from build123d import *

# Parameters (mm, degrees)
SKETCH1_W                    = 57.15
SKETCH1_H                    = 38.1
BASE_FLANGE1_DEPTH           = 1.89738
EDGE_FLANGE1_STRIP_W         = 11.38428
EDGE_FLANGE1_STRIP_H         = 1.89738
EDGE_FLANGE1_STRIP_CUT_DEPTH = 57.15
EDGE_FLANGE1_DEPTH           = 57.15
F_1_4_CLEARANCE_HOLE1_D      = 6.7564
F_1_4_CLEARANCE_HOLE2_D      = 6.7564
FILLET1_R                    = 6.35


# Sheet-metal steps are written as plain solids
with BuildPart() as part:
    # Sketch1 → Base-Flange1 (new body)
    with BuildSketch(Plane(origin=(0, 0, 0), x_dir=(1, 0, 0), z_dir=(0, 1, 0))):
        with Locations((0, -19.05)):
            Rectangle(SKETCH1_W, SKETCH1_H)
    extrude(amount=BASE_FLANGE1_DEPTH)

    # Edge-Flange1 strip (across the edge) → Edge-Flange1 strip cut (cut)
    with BuildSketch(Plane(origin=(28.575, 1.89738, 0), x_dir=(0, 0, 1), z_dir=(-1, 0, 0))):
        with Locations((-1.89738, -0.94869)):
            Rectangle(EDGE_FLANGE1_STRIP_W, EDGE_FLANGE1_STRIP_H)
    extrude(amount=EDGE_FLANGE1_STRIP_CUT_DEPTH, mode=Mode.SUBTRACT)

    # Edge-Flange1 section (across the edge) → Edge-Flange1 (add)
    with BuildSketch(Plane(origin=(28.575, 1.89738, 0), x_dir=(0, 0, 1), z_dir=(-1, 0, 0))):
        with BuildLine():
            Line((0, 1.89738), (0, 36.20262))
            Line((0, 36.20262), (1.89738, 36.20262))
            Line((1.89738, 36.20262), (1.89738, 1.89738))
            ThreePointArc((1.89738, 1.89738), (2.453109736, 0.555729736), (3.79476, 0))
            Line((3.79476, 0), (3.79476, -1.89738))
            ThreePointArc((3.79476, -1.89738), (1.111459471, -0.785920529), (0, 1.89738))
        make_face()
    extrude(amount=EDGE_FLANGE1_DEPTH)

    # 1/4 Clearance Hole1 (through all)
    with Locations(Plane(origin=(0, 1.89738, 0), x_dir=(1, 0, 0), z_dir=(0, 1, 0))):
        with Locations((-15.875, -25.4), (15.875, -25.4)):
            Hole(F_1_4_CLEARANCE_HOLE1_D / 2)

    # 1/4 Clearance Hole2 (through all)
    with Locations(Plane.XY.offset(1.89738)):
        with Locations((-15.875, 25.4), (15.875, 25.4)):
            Hole(F_1_4_CLEARANCE_HOLE2_D / 2)

    # Fillet1
    fillet1_edges = [part.edges().sort_by_distance(p)[0] for p in [
        (28.575, 38.1, 0.94869),
        (-28.575, 38.1, 0.94869),
        (28.575, 0.94869, 38.1),
        (-28.575, 0.94869, 38.1),
    ]]
    fillet(fillet1_edges, radius=FILLET1_R)


solid = part.part
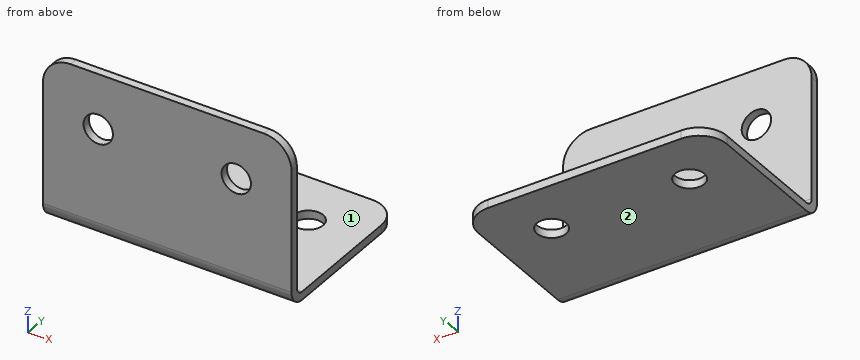
Read the model definition and answer for the solid it produces. Units are mm, in the model's axes. Face numbers are marked on the shaded views. A direction names the side the tool comes from. Round coordinates to 2 decimals unless told otherwise and drop trailing zeros. Order: outer loops, then holes, each group sorted by start corner. A loop starts at its lowest first (then second) coordinate and runs counter-clockwise, first axis right, second up.
1) For the marked faces 1 and 2, determine the directions among +Z, -Z, +X, -X, +Y, -Y from which every point of the face is accessible in a straight line to the end or side of a thin tool.
2) Flat-ended cylindrical pins translate along their axes: pin 1 (5 mm diameter, centred on x = 8, y = 29.5, fed in from +Z); pin 2 (4 mm diameter, centred on x = 21.5, z = 29.5, fed in from +Y). Find the tip coordinate at first contact, or state that the pin passes through.
3) Straight lines are drawn through the part: L1, parallel to Y at x = 12.5, z = 23; L2, parallel to Z at x = 0, y = 3. For each, find the intervals that lie inside material, in ascending order.
4) The part is cut by section C-C on x = 11.5. Write down the section's boundary in (y, z).
5) The part is cut by section A-A on y = 25.4. Write down the section's boundary in (x, z) (3 decimals).
6) The part is cut by section D-D on z = 19.5. Write down the section's boundary in (x, y) (3 decimals), plus the area to 3 significant figures.
Resolved:
1. face 1: +Z, +X, -X, +Y
1. face 2: -Z, +X, -X, +Y, -Y
2. pin 1: stops at z = 1.9
2. pin 2: stops at y = 1.9
3. L1: y = 0 to 1.9
3. L2: z = 0.08 to 2.07
4. outline: (0, 3.79) arc R3.79 ccw to (3.79, 0) - (38.1, 0) - (38.1, 1.9) - (3.79, 1.9) arc R1.9 cw to (1.9, 3.79) - (1.9, 38.1) - (0, 38.1) - close
5. outline: (-28.575, 0) - (-19.253, 0) - (-19.253, 1.897) - (-28.575, 1.897) - close; (-12.497, 0) - (12.497, 0) - (12.497, 1.897) - (-12.497, 1.897) - close; (19.253, 0) - (28.575, 0) - (28.575, 1.897) - (19.253, 1.897) - close
6. outline: (-28.575, 0) - (28.575, 0) - (28.575, 1.897) - (-28.575, 1.897) - close
6. area: 108 mm2
